```python
from build123d import *

# Parameters (mm, degrees)
BOSS_EXTRUDE1_DEPTH      = 8
BOSS_EXTRUDE1_DEPTH_BACK = 2
SKETCH1_R                = 1.5
SKETCH2_R                = 1.5
BOSS_EXTRUDE2_DEPTH      = 2
SKETCH5_R                = 1.5
BOSS_EXTRUDE3_DEPTH      = 2


with BuildPart() as part:
    # Sketch1 → Boss-Extrude1 (new, two sides: drawn at the far end of the back side and taken through both)
    with BuildSketch(Plane(origin=(0, 0, 0), x_dir=(1, 0, 0), z_dir=(0, 1, 0)).offset(-BOSS_EXTRUDE1_DEPTH_BACK)):
        with Locations(Location((-11.29860715, -4.069786589, 0), (0, 0, 270))):
            Circle(SKETCH1_R)
    extrude(amount=BOSS_EXTRUDE1_DEPTH + BOSS_EXTRUDE1_DEPTH_BACK)



with BuildPart() as body_2:
    # Sketch2 → Boss-Extrude2 (new body)
    with BuildSketch(Plane.XZ.offset(2)):
        Polygon((-14.106389898, 5.552921571), (-13.986931095, 2.379742892), (-11.179148348, 0.89660791), (-8.490824402, 2.586651607), (-8.610283205, 5.759830286), (-11.418065953, 7.242965268), align=None)
        with Locations(Location((-11.29860715, 4.069786589, 0), (0, 0, 90))):
            Circle(SKETCH2_R, mode=Mode.SUBTRACT)
    extrude(amount=BOSS_EXTRUDE2_DEPTH)


with BuildPart() as part_1:
    add(part.part)

    add(body_2.part)  # Boss-Extrude3 merges body 2
    # Sketch5 → Boss-Extrude3 (add)
    with BuildSketch(Plane.XZ.offset(4)):
        with Locations(Location((-11.29860715, 4.069786589, 0), (0, 0, 90))):
            Circle(SKETCH5_R)
    extrude(amount=-BOSS_EXTRUDE3_DEPTH)


solid = part_1.part
```
The model under review builds one solid part; all positions refer to its coordinate system, in mm. A direction names the side the tool comes from. Round coordinates to 2 decimals unless told otherwise and drop trailing zeros. Loops run counter-clockwise (first coordinate to the right, second up) from the corner with the lowest first, then second, coordinate; pieces in that order, holes last.
1) Tool access review of faces 1 (the face through (-11, 8, 4)), 2 (the face through (-11, -2, 6)): name each direction out of +Z, -Z, +X, -X, +Y, -Y from which nothing blocks a thin tool from reaching the whole face with its end or side.
Values follow:
face 1: +Z, -Z, +X, -X, +Y
face 2: +Y
2) Consider section D-D on z = 6. State the section outline as (x, y) points.
Values follow:
outline: (-13.4, -4) - (-9.06, -4) - (-9.06, -2) - (-13.4, -2) - close
3) Consider section C-C on y = 2. State the section outline as (x, z) points.
Values follow:
outline: circle Ø3 at (-11.3, 4.07)
4) Wall thickness on line 1 along Y through (x, z) = (-9.1, 5.5); line 2 along X through (y, z) = (-1.5, 4); line 3 along Z through (x, y) = (-10.6, 7.25): over which ranges is each line inside the solid? List them lowest first.
Values follow:
line 1: y = -4 to -2
line 2: x = -12.8 to -9.8
line 3: z = 2.74 to 5.4
5) Consider section A-A on z = 3.25. State the section outline as (x, y) points, then the cut area to 3 significant figures.
Values follow:
outline: (-14.02, -4) - (-8.52, -4) - (-8.52, -2) - (-10.04, -2) - (-10.04, 8) - (-12.55, 8) - (-12.55, -2) - (-14.02, -2) - close
area: 36.1 mm2
6) Consider section B-B on x = -12.55. State the section outline as (y, z) points.
Values follow:
outline: (-4, 1.62) - (-2, 1.62) - (-2, 3.24) - (8, 3.24) - (8, 4.9) - (-2, 4.9) - (-2, 6.53) - (-4, 6.53) - close
7) Clearance check with a flat-ended pin moving along its axis: P1, Ø1.5, axis at x = -10.5, y = 1, coming from the +Z side. State where the tip first meets the part, or that it passes through.
Values follow:
P1: stops at z = 5.57
